Geometry: final body of the model. Coordinates: model frame, mm. A direction names the side the tool comes from. Round coordinates to 2 decimals unless told otherwise and drop trailing zeros. Loops run counter-clockwise (first coordinate to the right, second up) from the corner with the lowest first, then second, coordinate; pieces in that order, holes last. Notation, with made-up numbers: M 36,67.25 L 93,67.25 A18 cw 93,95.25 Z; hole C -17,-16 d11. An arc over 180 degrees is marked long. Answer as a JSON object with one key per item and string values.
Autodesk Inventor part; units mm, degrees
ref_plane "YZ Plane" through (0, 0, 0) normal (1, 0, 0) x (0, 1, 0)
ref_plane "XZ Plane" through (0, 0, 0) normal (0, 1, 0) x (-1, 0, 0)
ref_plane "XY Plane" through (0, 0, 0) normal (0, 0, 1) x (1, 0, 0)
ref_plane "Work Plane1" through (7.5537, -38.3367, 0) normal (0, 0, 1) x (1, 0, 0)
sketch "Sketch1" plane through (7.5537, -38.3367, 0) normal (0, 0, 1) x (1, 0, 0)
  line L0 (-7.5537, -44.8483) -> (5.0701, -44.8483)
  line L1 (5.0701, -44.8483) -> (5.0701, -27.232)
  arc A0 (5.0701, -23.0946) -> (5.0701, -27.232) centre (5.1463, -25.1633) ccw
  line L2 (5.0701, -23.0946) -> (5.0701, -1.832)
  arc A1 (5.0701, 2.3054) -> (5.0701, -1.832) centre (5.1463, 0.2367) ccw
  line L3 (5.0701, 2.3054) -> (5.0701, 23.568)
  arc A2 (5.0701, 27.7054) -> (5.0701, 23.568) centre (5.1463, 25.6367) ccw
  line L4 (5.0701, 27.7054) -> (5.0701, 38.3367)
  line L5 (-7.5537, 38.3367) -> (5.0701, 38.3367)
  line L6 (-7.5537, 38.3367) -> (-7.5537, -44.8483)
  line L7 (5.2225, -44.8483) -> (17.8463, -44.8483)
  line L8 (17.8463, 38.3367) -> (17.8463, -44.8483)
  line L9 (5.2225, 38.3367) -> (17.8463, 38.3367)
  line L10 (5.2225, 27.7054) -> (5.2225, 38.3367)
  arc A3 (5.2225, 23.568) -> (5.2225, 27.7054) centre (5.1463, 25.6367) ccw
  line L11 (5.2225, 2.3054) -> (5.2225, 23.568)
  arc A4 (5.2225, -1.832) -> (5.2225, 2.3054) centre (5.1463, 0.2367) ccw
  line L12 (5.2225, -23.0946) -> (5.2225, -1.832)
  arc A5 (5.2225, -27.232) -> (5.2225, -23.0946) centre (5.1463, -25.1633) ccw
  line L13 (5.2225, -44.8483) -> (5.2225, -27.232)
  line L14 (-96.4537, -34.2184) -> (-96.4537, -44.8483)
  line L15 (-7.5537, -44.8483) -> (-96.4537, -44.8483)
  line L16 (-7.5537, -32.2245) -> (-7.5537, -44.8483)
  line L17 (-18.185, -32.2245) -> (-7.5537, -32.2245)
  arc A6 (-22.3224, -32.2245) -> (-18.185, -32.2245) centre (-20.2537, -32.1483) ccw
  line L18 (-43.585, -32.2245) -> (-22.3224, -32.2245)
  arc A7 (-47.7224, -32.2245) -> (-43.585, -32.2245) centre (-45.6537, -32.1483) ccw
  line L19 (-68.985, -32.2245) -> (-47.7224, -32.2245)
  arc A8 (-73.1224, -32.2245) -> (-68.985, -32.2245) centre (-71.0537, -32.1483) ccw
  line L20 (-94.385, -32.2245) -> (-73.1224, -32.2245)
  arc A9 (-96.4537, -34.2184) -> (-94.385, -32.2245) centre (-96.4537, -32.1483) ccw
  line L21 (-96.4537, -19.4483) -> (-96.4537, -30.0782)
  arc A10 (-94.385, -32.0721) -> (-96.4537, -30.0782) centre (-96.4537, -32.1483) ccw
  line L22 (-94.385, -32.0721) -> (-73.1224, -32.0721)
  arc A11 (-68.985, -32.0721) -> (-73.1224, -32.0721) centre (-71.0537, -32.1483) ccw
  line L23 (-68.985, -32.0721) -> (-47.7224, -32.0721)
  arc A12 (-43.585, -32.0721) -> (-47.7224, -32.0721) centre (-45.6537, -32.1483) ccw
  line L24 (-43.585, -32.0721) -> (-22.3224, -32.0721)
  arc A13 (-18.185, -32.0721) -> (-22.3224, -32.0721) centre (-20.2537, -32.1483) ccw
  line L25 (-18.185, -32.0721) -> (-7.5537, -32.0721)
  line L26 (-7.5537, -19.4483) -> (-7.5537, -32.0721)
  line L27 (-7.5537, -19.4483) -> (-96.4537, -19.4483)
  line L28 (-7.5537, 38.3367) -> (17.8463, 38.3367)
  line L29 (17.8463, 38.3367) -> (17.8463, -44.8483)
  line L30 (17.8463, -44.8483) -> (-7.5537, -44.8483)
  line L31 (-7.5537, -44.8483) -> (-7.5537, 38.3367)
  line L32 (-96.4537, -19.4483) -> (-7.5537, -19.4483)
  line L33 (-7.5537, -19.4483) -> (-7.5537, -44.8483)
  line L34 (-7.5537, -44.8483) -> (-96.4537, -44.8483)
  line L35 (-96.4537, -44.8483) -> (-96.4537, -19.4483)
  circle A14 centre (5.1463, -25.1633) radius 2.0701
  circle A15 centre (5.1463, 0.2367) radius 2.0701
  circle A16 centre (-45.6537, -32.1483) radius 2.0701
  circle A17 centre (-20.2537, -32.1483) radius 2.0701
  circle A18 centre (-71.0537, -32.1483) radius 2.0701
  circle A19 centre (5.1463, 25.6367) radius 2.0701
extrude "Plate1" add sketch "Sketch1" along normal blind 3.175 contours L6 L5 L4 A2 L3 A1 L2 A0 L1 L0 | L15 L14 A9 L20 A8 L19 A7 L18 A6 L17 L6 | L1 A14 L13 L30 | L17 A17 L25 L6 | L13 A5 L12 A4 L11 A3 L10 L9 L8 L7 | L25 A13 L24 A12 L23 A11 L22 A10 L21 L27 L6 | L35 A10 L22 A18 L20 A9 | L2 A15 L12 A14 | L18 A16 L24 A17 | L3 A19 L11 A15 | L10 A19 L4 L28 | L19 A18 L23 A16
fillet "Corner Round1" radius 6.35 6 edges at (0, 0, 1.5875) (25.4, 0, 1.5875) (-88.9, -57.785, 1.5875) (-88.9, -83.185, 1.5875) (0, -57.785, 1.5875) (25.4, -83.185, 1.5875)
equation "\"BendRadius\" = Thickness"
equation "\"BendReliefWidth\" = Thickness"
equation "\"BendReliefDepth\" = 0.5 * Thickness"
equation "\"CornerReliefSize\" = 4 * Thickness"
equation "\"MinimumRemnant\" = 2 * Thickness"
equation "\"TransitionRadius\" = BendRadius"
equation "\"JacobiRadiusSize\" = BendRadius"
equation "\"GapSize\" = Thickness"
equation "\"d0\" = BendRadius"
properties part number "Bumper Holder"
1) Cut plane A-A on x = -63.5. Return the cut outline in (y, z) (3 decimals), and give its area (3 significant figures).
Geometry results:
{"outline": "M -83.185,0 L -72.555,0 L -72.555,3.175 L -83.185,3.175 Z; M -68.415,0 L -57.785,0 L -57.785,3.175 L -68.415,3.175 Z", "area": "67.5 mm2"}
2) First-contact query: pin 1 (10 mm diameter, centred on x = -37.5, y = -66, fed in from -Z). Flat tip, straight axial feed; report the tip coordinate or a pass-through.
Geometry results:
{"pin 1": "z = 0"}
3) Cut plane D-D on y = -54. Return the cut outline in (x, z) (3 decimals).
Geometry results:
{"outline": "M -0.541,0 L 25.4,0 L 25.4,3.175 L -0.541,3.175 Z"}
4) Cut plane C-C on z = 2.2. Return the cut outline in (x, y) (3 decimals), and give its area (3 significant figures).
Geometry results:
{"outline": "M -88.9,-76.835 A6.35 ccw -82.55,-83.185 L 19.05,-83.185 A6.35 ccw 25.4,-76.835 L 25.4,-6.35 A6.35 ccw 19.05,0 L 6.35,0 A6.35 ccw 0,-6.35 L 0,-51.435 A6.35 cw -6.35,-57.785 L -82.55,-57.785 A6.35 ccw -88.9,-64.135 Z; hole M -65.569,-70.561 A2.07 ccw -61.431,-70.561 A2.07 ccw long Z; hole M -40.169,-70.561 A2.07 ccw -36.031,-70.561 A2.07 ccw long Z; hole M -14.769,-70.561 A2.07 ccw -10.631,-70.561 A2.07 ccw long Z; hole C 12.7,-63.5 d4.14; hole C 12.7,-38.1 d4.14; hole C 12.7,-12.7 d4.14", "area": "4,260 mm2"}
5) Set-up query: faces 1 (the face through (-88.9, -70, 2)), 2 (the face through (0, -29, 2)). Return all of +Z, -Z, +X, -X, +Y, -Y with unobstructed straight access to the full face (end or side cutting, diameter ignored); none if empty.
Geometry results:
{"face 1": "+Z, -Z, -X, +Y, -Y", "face 2": "+Z, -Z, -X, +Y"}
6) Line query: probe 1 along X at (y, z) = (-41.5, 0.8); probe 2 along Y at (x, z) = (-16.5, 0.6) (3 decimals); probe 3 along X at (y, z) = (-13.5, 1.3). Output: solid intervals per line, ascending.
Geometry results:
{"probe 1": "0 to 25.4", "probe 2": "-83.185 to -57.785", "probe 3": "0 to 10.79, 14.61 to 25.4"}
7) Cut plane B-B on y = -38.1. Return the cut outline in (x, z) (3 decimals), and give its area (3 significant figures).
Geometry results:
{"outline": "M 0,0 L 10.63,0 L 10.63,3.175 L 0,3.175 Z; M 14.77,0 L 25.4,0 L 25.4,3.175 L 14.77,3.175 Z", "area": "67.5 mm2"}
